Answer from the drawing. Dimensions are ordinates in mm from the lowest x, y and z of the part. A direction names the side the tool comes from. Round coordinates to 2 decimals unless told otherwise and drop trailing zeros. Write each loop counter-clockwise with the first axis right and the second up, starting at its lowest first coordinate (ties: lowest second). Pieces come first, ordered by that corner, then holes.
1. Find section C-C (x = 63.5). Write down the section's boundary in (y, z), and give its area (3 significant figures).
2. Straight lines are drawn through the part: probe 1 along Y at (x, z) = (63, 6); probe 2 along X at (y, z) = (82, 7); probe 3 along Y at (x, z) = (56, 45). For each, find the intervals that lie inside material, in ascending order.
3. Find section A-A (y = 82.55). Write down the section's boundary in (x, z).
4. Find section B-B (z = 5). Write down the section's boundary in (x, y).
5. Determine the mould class of the marked faces 5, 6 and 7 for opening direction X: pulls with the +X half, pulls with the -X half, needs draft (parallel to the pull), parting line crosses it, or undercut.
6. Find section D-D (z = 53). Write down the section's boundary in (x, y), and give its area (3 significant figures).
7. A tool of negligible diameter and unlimited length cuts with its end or side. For the marked faces 1, 2, 3 and 4, from which of +Z, -Z, +X, -X, +Y, -Y can it reach the whole face along a straight path? Write none if from no direction.
8. Flat-ended cylindrical pins translate along their axes: pin 1 Ø8 at (x, z) = (21, 20) entering from -Y; pin 2 Ø1.5 at (x, z) = (19.5, 52) entering from +Y; pin 3 Ø6 at (x, y) = (32.5, 10) entering from +Z; pin 4 Ø20.5 at (x, y) = (38.5, 61.5) entering from +Z (1 decimal). Find the tip coordinate at first contact, or state that the pin passes through.
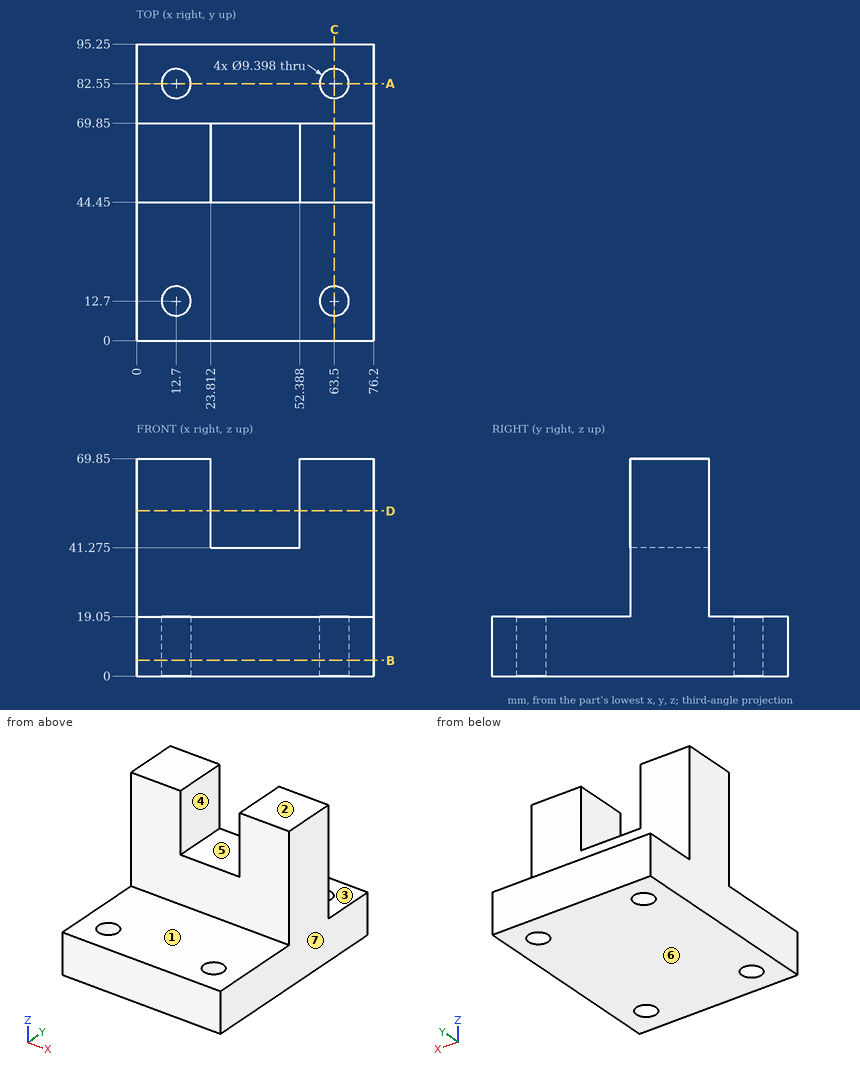
Worked answers:
1. outline: (0, 0) - (8, 0) - (8, 19.05) - (0, 19.05) - close; (17.4, 0) - (77.85, 0) - (77.85, 19.05) - (69.85, 19.05) - (69.85, 69.85) - (44.45, 69.85) - (44.45, 19.05) - (17.4, 19.05) - close; (87.25, 0) - (95.25, 0) - (95.25, 19.05) - (87.25, 19.05) - close
1. area: 2,750 mm2
2. probe 1: y = 0 to 8.03, 17.37 to 77.88, 87.22 to 95.25
2. probe 2: x = 0 to 8.03, 17.37 to 58.83, 68.17 to 76.2
2. probe 3: y = 44.45 to 69.85
3. outline: (0, 0) - (8, 0) - (8, 19.05) - (0, 19.05) - close; (17.4, 0) - (58.8, 0) - (58.8, 19.05) - (17.4, 19.05) - close; (68.2, 0) - (76.2, 0) - (76.2, 19.05) - (68.2, 19.05) - close
4. outline: (0, 0) - (76.2, 0) - (76.2, 95.25) - (0, 95.25) - close; hole circle Ø9.4 at (12.7, 12.7); hole circle Ø9.4 at (12.7, 82.55); hole circle Ø9.4 at (63.5, 12.7); hole circle Ø9.4 at (63.5, 82.55)
5. face 5: undercut
5. face 6: needs draft
5. face 7: pulls with the +X half
6. outline: (0, 44.45) - (23.81, 44.45) - (23.81, 69.85) - (0, 69.85) - close; (52.39, 44.45) - (76.2, 44.45) - (76.2, 69.85) - (52.39, 69.85) - close
6. area: 1,210 mm2
7. face 1: +Z, +X, -X, -Y
7. face 2: +Z, +X, -X, +Y, -Y
7. face 3: +Z, +X, -X, +Y
7. face 4: +Z, +Y, -Y
8. pin 1: stops at y = 0
8. pin 2: stops at y = 69.85
8. pin 3: stops at z = 19.05
8. pin 4: stops at z = 41.3
